```python
from build123d import *

# Parameters (mm, degrees)
F0_R     = 2
F1_DEPTH = 1.5
F0_W     = 50.8
F0_H     = 1.5
F2_DEPTH = 5
F3_DEPTH = 5
F4_W     = 50.8
F4_H     = 1.75
F5_DEPTH = 3
F7_DEPTH = 50.801


with BuildPart() as f1:
    # F0 (on Top) → F1 (new body)
    with BuildSketch(Plane.XY):
        Polygon((25.4, 24), (-25.4, 24), (0, 0), align=None)
        Polygon((-8.0304443836, 10.1160742342), (-8.0304443836, 22.0862291753), (8.0304443836, 22.0862291753), (8.0304443836, 10.1160742342), (0, 2.5282527694), align=None, mode=Mode.SUBTRACT)
        with Locations((-13.1485247985, 16.1011517048)):
            Circle(F0_R, mode=Mode.SUBTRACT)
        with Locations((12.2514752015, 16.1011517048)):
            Circle(F0_R, mode=Mode.SUBTRACT)
        Polygon((0, 0), (-25.4, 24), (-25.4, -24), align=None)
        Polygon((-23.3999999466, 19.3586534352), (-2.9120917277, 0), (-23.3999999466, -19.3586534352), align=None, mode=Mode.SUBTRACT)
        Polygon((0, 0), (-25.4, -24), (25.4, -24), align=None)
        Polygon((20.3712416834, -22), (-20.3712416834, -22), (0, -2.7515826614), align=None, mode=Mode.SUBTRACT)
        Polygon((25.4, -24), (25.4, 24), (0, 0), align=None)
        Polygon((23.4, -19.3586535591), (2.91209165, 0), (23.4, 19.3586535591), align=None, mode=Mode.SUBTRACT)
    extrude(amount=F1_DEPTH)

    # F0 (on Top) → F2 (join)
    with BuildSketch(Plane.XY):
        with Locations((0, -24.75)):
            Rectangle(F0_W, F0_H)
    extrude(amount=F2_DEPTH)

    # F0 (on Top) → F3 (join)
    with BuildSketch(Plane.XY):
        with Locations((0, 24.75)):
            Rectangle(F0_W, F0_H)
    extrude(amount=F3_DEPTH)

    # F4 (on face) → F5 (join)
    with BuildSketch(Plane.XZ.offset(-24)):
        with Locations((0, 4.125)):
            Rectangle(F4_W, F4_H)
    extrude(amount=F5_DEPTH)

    # F6 (on face) → F7 (cut, through all)
    with BuildSketch(Plane(origin=(-25.4, 0, 0), x_dir=(0, -1, 0), z_dir=(-1, 0, 0))):
        with BuildLine():
            ThreePointArc((-24, 1.5), (-23.375, 0.875), (-22.75, 1.5))
            Line((-22.75, 1.5), (-24, 1.5))
        make_face()
    extrude(amount=-F7_DEPTH, mode=Mode.SUBTRACT)


solid = f1.part
```
Input: part model. Units: mm. Frame: model coordinates. A direction names the side the tool comes from. Round coordinates to 2 decimals unless told otherwise and drop trailing zeros. Order: outer loops, then holes, each group sorted by start corner. A loop starts at its lowest first (then second) coordinate and runs counter-clockwise, first axis right, second up. Notation, with made-up numbers: (-28.5, 80) - (30.5, 80) arc R31 cw to (30.5, 115) - close; hole circle Ø11 at (12, 12). An arc over 180 degrees is marked (long way). One line per question, with ' | ' between items. Start each with the question number.
1) Contact query for flat-ended pins moving along their axis: P1, Ø8, axis at x = 9.5, y = 10.5, coming from the +Z side; P2, Ø1, axis at y = -1.5, z = 3, coming from the -X side. Output: stop coordinate, or through.
2) Cut plane A-A, the plane z = 3.95. Return the cut outline in (x, y).
3) Ray query, probe 1 along Y at (x, z) = (18, 2.6); probe 2 along Z at (x, y) = (-19, 22.5); probe 3 along Y at (x, z) = (-16.5, 1.05). Return the intervals inside material, ascending.
4) Cut plane D-D, the plane y = -10. Return the cut outline in (x, z), then the cut area to 3 significant figures.
5) Set-up query: faces 1 (the flat face through (0, -25, 5)), 2 (the flat face through (-23.4, 0, 1)), 3 (the flat face through (0, -24, 3)), 4 (the flat face through (0, 24, 2)). Return all of +Z, -Z, +X, -X, +Y, -Y with unobstructed straight access to the full face (end or side cutting, diameter ignored); none if empty.
6) Pull-direction query (Z, two-part tool) for faces 5 (the flat face through (0, 23, 5)), 6 (the flat face through (0, 23, 3.25)), 7 (the flat face through (0, 21, 4)); classes: +Z half, -Z half, draft (parallel to the pull), parting line (faces both ways), or undercut.
7) Cut plane B-B, the plane x = 5. Return the cut outline in (y, z) (3 decimals), then the cut area to 3 significant figures.
8) Cut plane C-C, the plane y = 11. Return the cut outline in (x, z), then the cut area to 3 significant figures.
Worked out:
1) P1: stops at z = 1.5 | P2: passes through
2) outline: (-25.4, -25.5) - (25.4, -25.5) - (25.4, -24) - (-25.4, -24) - close; (-25.4, 21) - (25.4, 21) - (25.4, 25.5) - (-25.4, 25.5) - close
3) probe 1: y = -25.5 to -24, 24 to 25.5 | probe 2: z = 0 to 1.5, 3.25 to 5 | probe 3: y = -25.5 to -22, -18.34 to -12.84, 12.84 to 22.94, 23.81 to 25.5
4) outline: (-25.4, 0) - (-23.4, 0) - (-23.4, 1.5) - (-25.4, 1.5) - close; (-13.5, 0) - (-7.67, 0) - (-7.67, 1.5) - (-13.5, 1.5) - close; (7.67, 0) - (13.5, 0) - (13.5, 1.5) - (7.67, 1.5) - close; (23.4, 0) - (25.4, 0) - (25.4, 1.5) - (23.4, 1.5) - close | area: 23.5 mm^2
5) face 1: +Z, +X, -X, +Y, -Y | face 2: +Z, -Z | face 3: +Z, +X, -X | face 4: +X, -X
6) face 5: +Z half | face 6: undercut | face 7: draft
7) outline: (-25.5, 0) - (-22, 0) - (-22, 1.5) - (-24, 1.5) - (-24, 5) - (-25.5, 5) - close; (-7.476, 0) - (-1.973, 0) - (-1.973, 1.5) - (-7.476, 1.5) - close; (1.973, 0) - (7.253, 0) - (7.253, 1.5) - (1.973, 1.5) - close; (21, 3.25) - (24, 3.25) - (24, 1.5) arc R0.625 cw to (22.75, 1.5) - (22.086, 1.5) - (22.086, 0) - (25.5, 0) - (25.5, 5) - (21, 5) - close | area: 41.7 mm^2
8) outline: (-25.4, 0) - (-23.4, 0) - (-23.4, 1.5) - (-25.4, 1.5) - close; (-14.55, 0) - (-8.03, 0) - (-8.03, 1.5) - (-14.55, 1.5) - close; (8.03, 0) - (14.55, 0) - (14.55, 1.5) - (8.03, 1.5) - close; (23.4, 0) - (25.4, 0) - (25.4, 1.5) - (23.4, 1.5) - close | area: 25.6 mm^2
